from build123d import *

# Parameters (mm, degrees)
PAD015_DEPTH         = 15
POCKET012_DEPTH      = 187.2426560764
POCKET012_DEPTH_BACK = 247.2426560764
SKETCH035_W          = 4
SKETCH035_H          = 14.6188021535
POCKET014_DEPTH      = 25
SKETCH040_W          = 56
SKETCH040_H          = 15
POCKET020_DEPTH      = 56
PAD021_DEPTH         = 15


with BuildPart() as part:
    # Sketch027 → Pad015 (new body, symmetric)
    with BuildSketch(Plane.YZ):
        with BuildLine():
            Line((-15, 6), (-15, -12.5))
            Line((-15, -12.5), (-11, -12.5))
            ThreePointArc((-7, -16.5), (-8.1715728753, -13.6715728753), (-11, -12.5))
            Line((-7, -16.5), (-7, -31.5))
            ThreePointArc((-11, -35.5), (-8.1715728753, -34.3284271247), (-7, -31.5))
            Line((-15, -35.5), (-11, -35.5))
            Line((-15, -35.5), (-15, -54))
            Line((-5, -54), (-15, -54))
            Line((0, 0), (-5, -54))
            Line((0, 0), (22, 0))
            ThreePointArc((26.8296291314, -3.7059047745), (25.043807145, -1.0332332985), (22, 0))
            Line((26.8296291314, -3.7059047745), (40.3058913312, -54))
            Line((50.3058913312, -54), (40.3058913312, -54))
            Line((50.3058913312, -54), (35.4205328152, 1.5529142706))
            ThreePointArc((35.4205328152, 1.5529142706), (33.2775464315, 4.7601200417), (29.6249778574, 6))
            Line((29.6249778574, 6), (-15, 6))
        make_face()
    extrude(amount=PAD015_DEPTH, both=True)

    # Sketch033 → Pocket012 (cut, two sides)
    with BuildSketch(Plane.XY.offset(-54)) as pocket012_sk:
        Polygon((-15, -11), (-15, -15), (-7.3094010768, -15), (-5, -11), align=None)
    pocket012 = extrude(amount=-POCKET012_DEPTH, mode=Mode.SUBTRACT) + extrude(pocket012_sk.sketch, amount=POCKET012_DEPTH_BACK, mode=Mode.SUBTRACT)

    # Mirrored004: Pocket012 across YZ
    add(pocket012.mirror(Plane.YZ), mode=Mode.SUBTRACT)

    # Sketch035 (on Face11 of Mirrored004) → Pocket014 (cut)
    with BuildSketch(Plane.YX.offset(-6)):
        with Locations((-13, 0)):
            Rectangle(SKETCH035_W, SKETCH035_H)
    extrude(amount=POCKET014_DEPTH, mode=Mode.SUBTRACT)

    # Sketch040 (on Face7 of Pocket014) → Pocket020 (cut)
    with BuildSketch(Plane(origin=(0, 0, 6), x_dir=(0, -1, 0), z_dir=(0, 0, 1))):
        with Locations((-22.3058913312, 0)):
            Rectangle(SKETCH040_W, SKETCH040_H)
    extrude(amount=-POCKET020_DEPTH, mode=Mode.SUBTRACT)

    # Sketch042 (on Face6 of Pocket020) → Pad021 (join)
    with BuildSketch(Plane(origin=(7.5, 0, 0), x_dir=(0, 1, 0), z_dir=(-1, 0, 0))):
        with BuildLine():
            Line((26.8296291314, 3.7059047745), (35.4205328152, -1.5529142706))
            ThreePointArc((29.6249778574, -6), (33.2775464315, -4.7601200417), (35.4205328152, -1.5529142706))
            Line((22, 0), (29.6249778574, -6))
            ThreePointArc((22, 0), (25.043807145, 1.0332332985), (26.8296291314, 3.7059047745))
        make_face()
        Polygon((34.325957072, 31.6825815187), (31.7377666209, 22.0233232558), (41.0678936399, 19.5233232558), (43.6560840909, 29.1825815187), align=None)
    extrude(amount=PAD021_DEPTH)


with BuildPart() as part_1:
    # Body014 placement: moved
    add(part.part.moved(Location((-22, 0, 0))))


solid = part_1.part
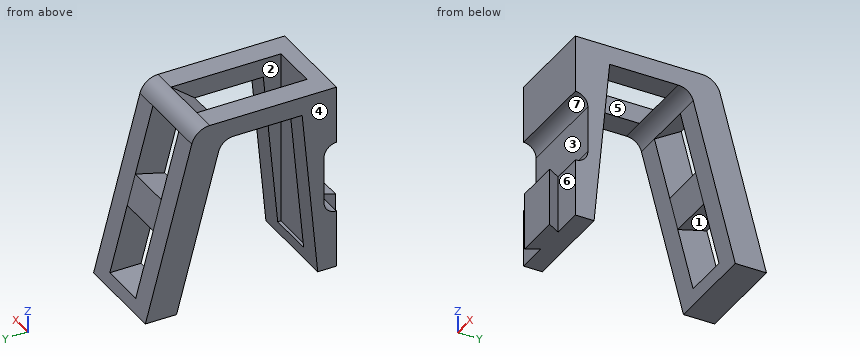
Verification items for the finished model (mm, model axes). Face numbers are marked on the shaded views. A direction names the side the tool comes from. Give positions to 0.01 mm unless a question says otherwise; leave off trailing zeros. Write each loop counter-clockwise with the first axis right and the second up, starting at its lowest first coordinate (ties: lowest second). Pieces come first, ordered by that corner, then holes. Notation, with made-up numbers: M 72,-26.75 L 85,-26.75 A32 ccw 85,10.25 Z; hole C -27,10 d4. An arc over 180 degrees is marked long. Write item = value, one per line.
(1) Access from +Z, -Z, +X, -X, +Y, -Y to the whole of each face (thin tool, end or side, straight path). Record for the marked faces 5, 6 and 7.
Found:
face_5 = +Z
face_6 = +Z, -Z, +X
face_7 = +X, -X, -Y
(2) Sectioned sample at D-D (x = -34.75). Record the cut outline in (y, z), then the cut area to 3 significant figures.
Found:
outline = M -11,-54 L -5,-54 L 0,0 L 22,0 A5 cw 26.83,-3.71 L 40.31,-54 L 50.31,-54 L 35.42,1.55 A6 ccw 29.62,6 L -11,6 L -11,-12.5 A4 cw -7,-16.5 L -7,-31.5 A4 cw -11,-35.5 Z
area = 1,190 mm2
(3) Go/stop test with flat-tipped pins: pin 1 Ø3 at (x, z) = (-9.5, -48) entering from -Y; pin 2 Ø7.5 at (x, z) = (-20.5, -25) entering from +Y; pin 3 Ø4 at (x, y) = (-26, 14.5) entering from +Z; pin 4 Ø8 at (x, y) = (-9.5, 14.5) entering from -Z. Record where each tip stops, or that it passes through.
Found:
pin_1 = -11
pin_2 = 43.54
pin_3 = through
pin_4 = 0
(4) Sectioned sample at B-B (x = -19.25). Record the cut outline in (y, z), then the cut area to 3 significant figures.
Found:
outline = M -15,-54 L -5,-54 L -4.63,-50 L -5.69,-50 L -5.69,6 L -11,6 L -11,-12.5 A4 cw -7,-16.5 L -7,-31.5 A4 cw -11,-35.5 L -15,-35.5 Z; M 22,0 A5 cw 26.83,-3.71 L 35.42,1.55 A6 ccw 29.62,6 Z; M 31.74,-22.02 L 34.33,-31.68 L 43.66,-29.18 L 41.07,-19.52 Z; M 39.23,-50 L 40.31,-54 L 50.31,-54 L 49.23,-50 Z
area = 512 mm2
(5) Material ranges on line 1 (X direction, y = 47, z = -47.5); line 2 (Z direction, x = -9.5, y = 20); line 3 (Y direction, x = -18, z = -27), recorded low to high.
Found:
line_1 = -37 to -29.5, -14.5 to -7
line_2 = 0 to 6
line_3 = -7 to -5.69, 33.07 to 43.07
(6) Sectioned sample at C-C (z = -11). Record the cut outline in (x, y).
Found:
outline = M -37,-11 L -7,-11 L -7,-1.02 L -14.5,-1.02 L -14.5,-5.69 L -29.5,-5.69 L -29.5,-1.02 L -37,-1.02 Z; M -37,28.78 L -29.5,28.78 L -29.5,38.78 L -37,38.78 Z; M -14.5,28.78 L -7,28.78 L -7,38.78 L -14.5,38.78 Z
(7) Draft check along Y on the marked faces 1, 2, 3 and 4. Enter one of: released by +Y, released by -Y, zero draft, split by the parting line, or undercut.
Found:
face_1 = released by +Y
face_2 = undercut
face_3 = released by -Y
face_4 = zero draft
(8) Sectioned sample at A-A (y = 13). Record the cut outline in (x, z), then the cut area to 3 significant figures.
Found:
outline = M -37,0 L -29.5,0 L -29.5,6 L -37,6 Z; M -14.5,0 L -7,0 L -7,6 L -14.5,6 Z
area = 90.0 mm2
